from build123d import *

# Parameters (mm, degrees)
BOSS_EXTRUDE1_DEPTH     = 0.79375
FILLET1_R               = 19.05
CUT_EXTRUDE1_DEPTH      = 80.251873253
CUT_EXTRUDE1_DEPTH_BACK = 80.251873253
SKETCH2_W               = 12.7
SKETCH2_H               = 6.35
FILLET2_R               = 1.5875
CHAMFER1_SIZE           = 5.08
FILLET3_R               = 3.175


with BuildPart() as part:
    # Sketch1 → Boss-Extrude1 (new, symmetric)
    with BuildSketch(Plane(origin=(0, 0, 0), x_dir=(1, 0, 0), z_dir=(0, 1, 0))):
        Polygon((-46.83125, 58.7375), (-46.83125, 0), (46.83125, 0), (46.83125, 58.7375), (53.18125, 58.7375), (53.18125, -15.875), (-53.18125, -15.875), (-53.18125, 58.7375), align=None)
    extrude(amount=BOSS_EXTRUDE1_DEPTH, both=True)

    # Fillet1
    fillet1_edges = [part.edges().sort_by_distance(p)[0] for p in [
        (53.18125, 0, 15.875),
        (-53.18125, 0, 15.875),
    ]]
    fillet(fillet1_edges, radius=FILLET1_R)

    # Sketch2 → Cut-Extrude1 (cut, two sides: drawn at the far end of the back side and taken through both)
    with BuildSketch(Plane(origin=(0, 0.79375, 0), x_dir=(1, 0, 0), z_dir=(0, 1, 0)).offset(-CUT_EXTRUDE1_DEPTH_BACK)):
        with Locations((0, -7.9375)):
            Rectangle(SKETCH2_W, SKETCH2_H)
    extrude(amount=CUT_EXTRUDE1_DEPTH + CUT_EXTRUDE1_DEPTH_BACK, mode=Mode.SUBTRACT)

    # Fillet2
    fillet2_edges = [part.edges().sort_by_distance(p)[0] for p in [
        (6.35, 0, 4.7625),
        (6.35, 0, 11.1125),
        (-6.35, 0, 11.1125),
        (-6.35, 0, 4.7625),
    ]]
    fillet(fillet2_edges, radius=FILLET2_R)

    # Chamfer1
    chamfer1_edges = [part.edges().sort_by_distance(p)[0] for p in [
        (-53.18125, 0, -58.7375),
        (53.18125, 0, -58.7375),
    ]]
    chamfer(chamfer1_edges, length=CHAMFER1_SIZE)

    # Fillet3
    fillet3_edges = [part.edges().sort_by_distance(p)[0] for p in [
        (-46.83125, 0, 0),
        (46.83125, 0, 0),
    ]]
    fillet(fillet3_edges, radius=FILLET3_R)


solid = part.part
Can you work these out from the model? Positions are in its coordinate system, mm. A direction names the side the tool comes from. Round coordinates to 2 decimals unless told otherwise and drop trailing zeros. Write each loop counter-clockwise with the first axis right and the second up, starting at its lowest first coordinate (ties: lowest second). Pieces come first, ordered by that corner, then holes. Notation, with made-up numbers: M -29.5,38.5 L 17.5,38.5 A9 ccw 17.5,43.5 Z; hole C 7.5,38.5 d6. An arc over 180 degrees is marked long. Use a Markdown table: item, result.
Item 1: We'd pull the mould along X, two halves only. Please class faces 1 (the face through (50.61, 0.01, -56.23)), 2 (the face through (-45.88, -0.01, -0.91)), 3 (the face through (-4, 0.794, 1)): released by +X, released by -X, zero draft, split by the parting line, or undercut.
Found:
| item | result |
|---|---|
| face 1 | released by +X |
| face 2 | undercut |
| face 3 | zero draft |
Item 2: I want a section at D-D (x = -39). List the corners of the cut face in (y, z) for me, and give its area (3 significant figures).
Found:
| item | result |
|---|---|
| outline | M -0.79,0 L 0.79,0 L 0.79,15.24 L -0.79,15.24 Z |
| area | 24.2 mm2 |
Item 3: If I drill on line 1 along X through (y, z) = (0.1, -29.5); line 2 along Z through (x, y) = (-11, -0.5) (3 decimals); line 3 along X through (y, z) = (-0.55, 7.5), over which ranges is the centre line in solid material (lowest first)? Write a range as [from, to].
Found:
| item | result |
|---|---|
| line 1 | x = [-53.18, -46.83], [46.83, 53.18] |
| line 2 | z = [0, 15.875] |
| line 3 | x = [-49.91, -6.35], [6.35, 49.91] |
Item 4: Which directions (+Z, -Z, +X, -X, +Y, -Y) give clear straight access to the entire face, cutting with the end or side of a thin tool? Please do faces 4 (the face through (-4, -0.794, 1)), 5 (the face through (45.926, -0.011, -0.955)).
Found:
| item | result |
|---|---|
| face 4 | +Z, -Z, +X, -X, -Y |
| face 5 | -Z, +Y, -Y |
Item 5: For pin 1 Ø0.8 at (y, z) = (-0.5, 8.5) entering from +X; pin 2 Ø0.5 at (y, z) = (0, 8.5) entering from -X (3 decimals), each with a flat end and sliding along its axis, tell me the tip position at first contact or that it passes through.
Found:
| item | result |
|---|---|
| pin 1 | stops at x = 49.49 |
| pin 2 | stops at x = -49.375 |
Item 6: I want a section at C-C (x = -14.5). List the corners of the cut face in (y, z) for me (3 decimals), and give its area (3 significant figures).
Found:
| item | result |
|---|---|
| outline | M -0.794,0 L 0.794,0 L 0.794,15.875 L -0.794,15.875 Z |
| area | 25.2 mm2 |
Item 7: I want a section at B-B (z = -7.5). List the corners of the cut face in (x, y) for me.
Found:
| item | result |
|---|---|
| outline | M -53.18,-0.79 L -46.83,-0.79 L -46.83,0.79 L -53.18,0.79 Z; M 46.83,-0.79 L 53.18,-0.79 L 53.18,0.79 L 46.83,0.79 Z |
